Design review of the part built by this model. Coordinates are the model's own, in mm. Face numbers are marked on the shaded views. A direction names the side the tool comes from. Coordinates: 2 decimals unless noted, no trailing zeros. Order: outer loops, then holes, each group sorted by start corner. A loop starts at its lowest first (then second) coordinate and runs counter-clockwise, first axis right, second up. Notation, with made-up numbers: M 86.25,-32 L 138.25,-32 A32 ccw 138.25,0 Z; hole C 79.5,-15.75 d8. An arc over 180 degrees is marked long. Answer as a JSON object with one key per item and string values.
from build123d import *

# Parameters (mm, degrees)
F1_DEPTH = 27
F2_DEPTH = 15
F3_R     = 1


with BuildPart() as f1:
    # F0 (on Top) → F1 (new body)
    with BuildSketch(Plane.XY):
        Polygon((-10.4, 0.75), (-13, 0.75), (-13, -0.75), (-10.4, -0.75), (10.4, -0.75), (13, -0.75), (13, 0.75), (10.4, 0.75), align=None)
    extrude(amount=F1_DEPTH)

    # F0 (on Top) → F2 (join)
    with BuildSketch(Plane.XY):
        Polygon((-13, 1.4), (-13, 0.75), (-10.4, 0.75), align=None)
        Polygon((-10.4, -0.75), (-13, -0.75), (-13, -1.4), align=None)
        Polygon((13, 1.4), (10.4, 0.75), (13, 0.75), align=None)
        Polygon((13, -0.75), (10.4, -0.75), (13, -1.4), align=None)
    extrude(amount=F2_DEPTH)

    # F3
    f3_edges = [f1.edges().sort_by_distance(p)[0] for p in [
        (-13, 0, 27),
        (13, 0, 27),
    ]]
    fillet(f3_edges, radius=F3_R)


solid = f1.part
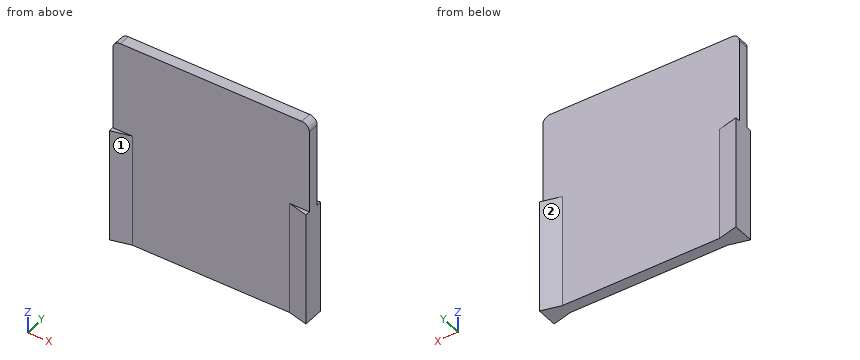
1) Add section C-C (z = 25). State the section outline as (x, y) points, and give its area (3 significant figures).
Taken from the geometry:
{"outline": "M -13,-0.75 L 13,-0.75 L 13,0.75 L -13,0.75 Z", "area": "39.0 mm2"}
2) Insertion check: pin 1 Ø1 at (x, y) = (-1, 0) entering from -Z; pin 2 Ø10 at (x, z) = (2.5, 21) entering from -Y; pin 3 Ø1 at (x, z) = (9, 8) entering from +Y. Each pin has a flat end and moves straight along its axis. Give the tip position at first contact, or say it passes through.
Taken from the geometry:
{"pin 1": "stops at z = 0", "pin 2": "stops at y = -0.75", "pin 3": "stops at y = 0.75"}
3) Add section B-B (x = -4). State the section outline as (y, z) points.
Taken from the geometry:
{"outline": "M -0.75,0 L 0.75,0 L 0.75,27 L -0.75,27 Z"}
4) To check wall thickness, follow L1, parallel to Y at x = 5.75, z = 15.5. State the ranges of the line that lie inside material, in increasing order.
Taken from the geometry:
{"L1": "y = -0.75 to 0.75"}
5) Add section A-A (z = 4.5). State the section outline as (x, y) points.
Taken from the geometry:
{"outline": "M -13,-1.4 L -10.4,-0.75 L 10.4,-0.75 L 13,-1.4 L 13,1.4 L 10.4,0.75 L -10.4,0.75 L -13,1.4 Z"}
6) Tool access review of the marked faces 1 and 2: name each direction out of +Z, -Z, +X, -X, +Y, -Y from which nothing blocks a thin tool from reaching the whole face with its end or side.
Taken from the geometry:
{"face 1": "+Z, -Z, -Y", "face 2": "+Z, -Z, +Y"}
